```python
from build123d import *

# Parameters (mm, degrees)
SKETCH_1_R          = 8
EXTRUDE_1_DEPTH     = 0.65
EXTRUDE_START       = 0.65
SKETCH_2_R          = 6.05
SKETCH_2_R_2        = 5.1
EXTRUDE_2_DEPTH     = 0.85
CUT_EXTRUDE_START   = 0.65
SKETCH_3_R          = 5.1
CUT_EXTRUDE_1_DEPTH = 0.01
CUT_EXTRUDE_2_DEPTH = 0.64
CHAMFER_1_SIZE      = 0.3


with BuildPart() as part:
    # 草图1 → 凸台-拉伸1 (new body)
    with BuildSketch(Plane.XY):
        Circle(SKETCH_1_R)
    extrude(amount=EXTRUDE_1_DEPTH)

    # 草图2 → 凸台-拉伸2 (add)
    with BuildSketch(Plane.XY.offset(EXTRUDE_START)):
        Circle(SKETCH_2_R)
        Circle(SKETCH_2_R_2, mode=Mode.SUBTRACT)
    extrude(amount=EXTRUDE_2_DEPTH)

    # 草图3 → 切除-拉伸1 (cut)
    with BuildSketch(Plane.XY.offset(CUT_EXTRUDE_START)):
        Circle(SKETCH_3_R)
    extrude(amount=-CUT_EXTRUDE_1_DEPTH, mode=Mode.SUBTRACT)

    # 草图4 → 切除-拉伸2 (cut)
    with BuildSketch(Plane.XY):
        Polygon((3.675, 3.675), (3.675, -3.675), (-3.675, -3.675), (-3.675, 0), (-3.675, 3.675), align=None)
    extrude(amount=CUT_EXTRUDE_2_DEPTH, mode=Mode.SUBTRACT)

    # 倒角1
    chamfer_1_edges = [part.edges().sort_by_distance(p)[0] for p in [
        (-5.1, 0, 1.5),
    ]]
    chamfer(chamfer_1_edges, length=CHAMFER_1_SIZE)


solid = part.part
```
Verification items for the finished model (mm, model axes). A direction names the side the tool comes from. Give positions to 0.01 mm unless a question says otherwise; leave off trailing zeros. Write each loop counter-clockwise with the first axis right and the second up, starting at its lowest first coordinate (ties: lowest second). Pieces come first, ordered by that corner, then holes. Notation, with made-up numbers: (46.5, 31.5) - (58.5, 31.5) arc R24 cw to (58.5, 51.5) - close; hole circle Ø2 at (73, -39). An arc over 180 degrees is marked (long way). Put each result on its own line as item: value.
Q1. Section check D-D on y = -5.75. Record the cut outline in (x, z), and give its area (3 significant figures).
Result:
outline: (-5.56, 0) - (5.56, 0) - (5.56, 0.65) - (1.88, 0.65) - (1.88, 1.5) - (-1.88, 1.5) - (-1.88, 0.65) - (-5.56, 0.65) - close
area: 10.4 mm2
Q2. Set-up check for faces 1 (the face through (5, 0, 0)), 2 (the face through (2.4, -4.5, 0.9)): record each of +Z, -Z, +X, -X, +Y, -Y from which the full face is reachable in a straight line by a thin tool's end or side.
Result:
face 1: -Z, +X, -X, +Y, -Y
face 2: +Z
Q3. Scan lines: probe 1 along Y at (x, z) = (0, 1.1); probe 2 along Z at (x, y) = (7, 3.5); probe 3 along Y at (x, z) = (2.75, 1.3). Record each from-to range of solid material in increasing order. Write a range as from..to.
Result:
probe 1: -6.05..-5.1, 5.1..6.05
probe 2: 0..0.65
probe 3: -5.39..-4.41, 4.41..5.39
Q4. Section check A-A on y = 0. Record the cut outline in (x, z) (3 decimals), and give its area (3 significant figures).
Result:
outline: (-8, 0) - (-3.675, 0) - (-3.675, 0.64) - (-5.1, 0.64) - (-5.1, 1.2) - (-5.4, 1.5) - (-6.05, 1.5) - (-6.05, 0.65) - (-8, 0.65) - close; (3.675, 0) - (8, 0) - (8, 0.65) - (6.05, 0.65) - (6.05, 1.5) - (5.4, 1.5) - (5.1, 1.2) - (5.1, 0.64) - (3.675, 0.64) - close
area: 7.12 mm2
Q5. Section check C-C on z = 0.4. Record the cut outline in (x, y) (3 decimals).
Result:
outline: circle Ø16 at (0, 0); hole (-3.675, -3.675) - (3.675, -3.675) - (3.675, 3.675) - (-3.675, 3.675) - close
Q6. Depth check by flat-ended pin: P1, Ø1.1, axis at x = 1.5, y = 4.5, coming from the +Z side; P2, Ø1, axis at x = -0.5, y = -4, coming from the +Z side; P3, Ø1, axis at x = 0, y = -1.5, coming from the +Z side; P4, Ø0.5, axis at x = -0.5, z = 0.5, coming from the -Y side. Enter the tip coordinate at first touch or a pass-through.
Result:
P1: z = 1.39
P2: z = 0.64
P3: through
P4: y = -8
